```python
from build123d import *

# Parameters (mm, degrees)
SKETCH1_W           = 20.7
SKETCH1_H           = 15.5
BOSS_EXTRUDE1_DEPTH = 1.6
FILLET1_R           = 1
SKETCH2_R           = 0.75
SKETCH2_R_2         = 0.5
CUT_EXTRUDE1_DEPTH  = 14.028622337
SKETCH2_3_R         = 1
SKETCH2_3_R_2       = 0.75
SKETCH2_3_R_3       = 0.5
CUT_EXTRUDE3_DEPTH  = 0.05
CUT_EXTRUDE2_DEPTH  = 14.028622337
SKETCH4_W           = 2.5
SKETCH4_H           = 4.5
BOSS_EXTRUDE2_DEPTH = 0.78


with BuildPart() as part:
    # Sketch1 → Boss-Extrude1 (new body)
    with BuildSketch(Plane(origin=(0, 0, 0), x_dir=(1, 0, 0), z_dir=(0, 1, 0))):
        Rectangle(SKETCH1_W, SKETCH1_H)
    extrude(amount=BOSS_EXTRUDE1_DEPTH)

    # Fillet1
    fillet1_edges = [part.edges().sort_by_distance(p)[0] for p in [
        (10.35, 0.8, 7.75),
        (-10.35, 0.8, 7.75),
        (-10.35, 0.8, -7.75),
        (10.35, 0.8, -7.75),
    ]]
    fillet(fillet1_edges, radius=FILLET1_R)

    # Sketch2 → Cut-Extrude1 (cut, through all)
    with BuildSketch(Plane(origin=(0, 1.6, 0), x_dir=(1, 0, 0), z_dir=(0, 1, 0))):
        with Locations(Location((-6.25, -6.25, 0), (0, 0, 270))):
            Circle(SKETCH2_R)
        with Locations(Location((-3.75, -4.75, 0), (0, 0, 270))):
            Circle(SKETCH2_R_2)
        with Locations(Location((-1.25, -4.75, 0), (0, 0, 270))):
            Circle(SKETCH2_R_2)
        with Locations(Location((1.25, -4.75, 0), (0, 0, 270))):
            Circle(SKETCH2_R_2)
        with Locations(Location((3.75, -4.75, 0), (0, 0, 270))):
            Circle(SKETCH2_R_2)
        with Locations(Location((6.25, -6.25, 0), (0, 0, 270))):
            Circle(SKETCH2_R)
    cut_extrude1 = extrude(amount=-CUT_EXTRUDE1_DEPTH, mode=Mode.SUBTRACT)

    # Sketch2_3 → Cut-Extrude3 (cut)
    # profile 1 of 6: a face of its own
    with BuildSketch(Plane(origin=(0, 1.6, 0), x_dir=(1, 0, 0), z_dir=(0, 1, 0))):
        with Locations(Location((-6.25, -6.25, 0), (0, 0, 270))):
            Circle(SKETCH2_3_R)
        with Locations(Location((-6.25, -6.25, 0), (0, 0, 270))):
            Circle(SKETCH2_3_R_2, mode=Mode.SUBTRACT)
    # profile 2 of 6: a face of its own
    with BuildSketch(Plane(origin=(0, 1.6, 0), x_dir=(1, 0, 0), z_dir=(0, 1, 0))):
        with Locations(Location((-3.75, -4.75, 0), (0, 0, 270))):
            Circle(SKETCH2_3_R_2)
        with Locations(Location((-3.75, -4.75, 0), (0, 0, 270))):
            Circle(SKETCH2_3_R_3, mode=Mode.SUBTRACT)
    # profile 3 of 6: a face of its own
    with BuildSketch(Plane(origin=(0, 1.6, 0), x_dir=(1, 0, 0), z_dir=(0, 1, 0))):
        with Locations(Location((-1.25, -4.75, 0), (0, 0, 270))):
            Circle(SKETCH2_3_R_2)
        with Locations(Location((-1.25, -4.75, 0), (0, 0, 270))):
            Circle(SKETCH2_3_R_3, mode=Mode.SUBTRACT)
    # profile 4 of 6: a face of its own
    with BuildSketch(Plane(origin=(0, 1.6, 0), x_dir=(1, 0, 0), z_dir=(0, 1, 0))):
        with Locations(Location((1.25, -4.75, 0), (0, 0, 90))):
            Circle(SKETCH2_3_R_2)
        with Locations(Location((1.25, -4.75, 0), (0, 0, 270))):
            Circle(SKETCH2_3_R_3, mode=Mode.SUBTRACT)
    # profile 5 of 6: a face of its own
    with BuildSketch(Plane(origin=(0, 1.6, 0), x_dir=(1, 0, 0), z_dir=(0, 1, 0))):
        with Locations(Location((3.75, -4.75, 0), (0, 0, 90))):
            Circle(SKETCH2_3_R_2)
        with Locations(Location((3.75, -4.75, 0), (0, 0, 270))):
            Circle(SKETCH2_3_R_3, mode=Mode.SUBTRACT)
    # profile 6 of 6: a face of its own
    with BuildSketch(Plane(origin=(0, 1.6, 0), x_dir=(1, 0, 0), z_dir=(0, 1, 0))):
        with Locations(Location((6.25, -6.25, 0), (0, 0, 90))):
            Circle(SKETCH2_3_R)
        with Locations(Location((6.25, -6.25, 0), (0, 0, 270))):
            Circle(SKETCH2_3_R_2, mode=Mode.SUBTRACT)
    cut_extrude3 = extrude(amount=-CUT_EXTRUDE3_DEPTH, mode=Mode.SUBTRACT)

    # Mirror1: Cut-Extrude1, Cut-Extrude3 across plane
    add(cut_extrude1.mirror(Plane.XY), mode=Mode.SUBTRACT)
    add(cut_extrude3.mirror(Plane.XY), mode=Mode.SUBTRACT)

    # Sketch3 → Cut-Extrude2 (cut, through all)
    with BuildSketch(Plane(origin=(0, 1.6, 0), x_dir=(1, 0, 0), z_dir=(0, 1, 0))):
        with BuildLine():
            Line((-9.35, -4.25), (-9.35, 4.25))
            ThreePointArc((-9.35, 4.25), (-8.85, 4.75), (-8.35, 4.25))
            Line((-8.35, 4.25), (-8.35, -4.25))
            ThreePointArc((-8.35, -4.25), (-8.85, -4.75), (-9.35, -4.25))
        make_face()
    cut_extrude2 = extrude(amount=-CUT_EXTRUDE2_DEPTH, mode=Mode.SUBTRACT)

    # Mirror2: Cut-Extrude2 across plane
    add(cut_extrude2.mirror(Plane(origin=(0, 0, 0), x_dir=(0, 0, 1), z_dir=(1, 0, 0))), mode=Mode.SUBTRACT)

    # Sketch4 → Boss-Extrude2 (add)
    with BuildSketch(Plane(origin=(0, 1.6, 0), x_dir=(1, 0, 0), z_dir=(0, 1, 0))):
        Rectangle(SKETCH4_W, SKETCH4_H)
    extrude(amount=BOSS_EXTRUDE2_DEPTH)


solid = part.part
```
The model under review builds one solid part; all positions refer to its coordinate system, in mm. A direction names the side the tool comes from. Round coordinates to 2 decimals unless told otherwise and drop trailing zeros. Loops run counter-clockwise (first coordinate to the right, second up) from the corner with the lowest first, then second, coordinate; pieces in that order, holes last.
Item 1: Take a section at D-D (x = 8.85). Write out the cut boundary in (y, z), then the cut area to 3 significant figures.
Determined:
outline: (0, -7.75) - (1.6, -7.75) - (1.6, -4.75) - (0, -4.75) - close; (0, 4.75) - (1.6, 4.75) - (1.6, 7.75) - (0, 7.75) - close
area: 9.60 mm2
Item 2: Mouldability with a two-part tool opening along X and no side actions: class faces 1 (the face through (-6.2, 0.8, -5.5)), 2 (the face through (10.049, 0.811, 7.465)), 3 (the face through (0, 1, 7.75)) as released by +X, released by -X, zero draft, split by the parting line, or undercut.
Determined:
face 1: undercut
face 2: released by +X
face 3: zero draft
Item 3: Clearance check with a flat-ended pin moving along its axis: pin 1 Ø1.2 at (x, z) = (3.75, -4.75) entering from +Y. State where the tip first meets the part, or that it passes through.
Determined:
pin 1: stops at y = 1.55
Item 4: Take a section at C-C (z = -1.25). Write out the cut boundary in (x, y), then the cut area to 3 significant figures.
Determined:
outline: (-10.35, 0) - (-9.35, 0) - (-9.35, 1.6) - (-10.35, 1.6) - close; (-8.35, 0) - (8.35, 0) - (8.35, 1.6) - (1.25, 1.6) - (1.25, 2.38) - (-1.25, 2.38) - (-1.25, 1.6) - (-8.35, 1.6) - close; (9.35, 0) - (10.35, 0) - (10.35, 1.6) - (9.35, 1.6) - close
area: 31.9 mm2
Item 5: Take a section at B-B (y = 0.5). Give the number of separate pieces and of enclosed holes in the cut face, then the cut area to 3 significant figures.
Determined:
separate pieces: 1
enclosed holes: 14
area: 288 mm2
Item 6: For faces 4 (the face through (8.86, 0.81, -4.75)), 5 (the face through (0, 0, 0)), list the 3-axis set-ups (+Z, -Z, +X, -X, +Y, -Y) from which the entire face can be reached by the end or side of a thin tool; tool diameter is ignored.
Determined:
face 4: +Y, -Y
face 5: +Z, -Z, +X, -X, -Y
Item 7: Take a section at A-A (x = -3.75). Write out the cut boundary in (y, z).
Determined:
outline: (0, -7.75) - (1.6, -7.75) - (1.6, -5.5) - (1.55, -5.5) - (1.55, -5.25) - (0, -5.25) - close; (0, -4.25) - (1.55, -4.25) - (1.55, -4) - (1.6, -4) - (1.6, 4) - (1.55, 4) - (1.55, 4.25) - (0, 4.25) - close; (0, 5.25) - (1.55, 5.25) - (1.55, 5.5) - (1.6, 5.5) - (1.6, 7.75) - (0, 7.75) - close
Item 8: For line 1 (X direction, y = 0.9, z = 4); line 2 (Z direction, x = 1.5, y = 1.3); line 3 (X direction, y = 0.3, z = -6.5), list the stretches that pass through material, from the lowest coordinate up.
Determined:
line 1: x = -10.35 to -9.35, -8.35 to 8.35, 9.35 to 10.35
line 2: z = -7.75 to -5.18, -4.32 to 4.32, 5.18 to 7.75
line 3: x = -10.35 to -6.96, -5.54 to 5.54, 6.96 to 10.35
